Read the model definition and answer for the solid it produces. Units are mm, in the model's axes. Face numbers are marked on the shaded views. A direction names the side the tool comes from. Give positions to 0.01 mm unless a question says otherwise; leave off trailing zeros. Order: outer loops, then holes, each group sorted by start corner. A loop starts at its lowest first (then second) coordinate and runs counter-clockwise, first axis right, second up. Notation, with made-up numbers: (-9.75, -40) - (42.25, -40) arc R16 ccw to (42.25, -29) - close; hole circle Ø3 at (82.25, -33). An arc over 180 degrees is marked (long way). Use a Markdown table: item, result. Add a question column.
1. A cutting plane is placed at B-B on x = -22.5. Determine the outline of the cut face in (y, z), and give its area (3 significant figures).
2. A cutting plane is placed at A-A on y = -28. Determine the outline of the cut face in (x, z), and give its area (3 significant figures).
3. For a pull along X with two mould halves and no side action, classify the marked faces 3, 4, 5 and 6 as released by +X, released by -X, zero draft, split by the parting line, or undercut.
4. Which of the six approach directions +Z, -Z, +X, -X, +Y, -Y give full straight-line access (tool end or side, diameter ignored) to the marked faces 1 and 2?
5. Consider L1, parallel to Z at x = -32, y = -68; L2, parallel to X at y = -28, z = 5. Determine where each line is inside the solid, lowest interval first.
6. A cutting plane is placed at C-C on z = -3.5. Determine the outline of the cut face in (x, y), and give its area (3 significant figures).
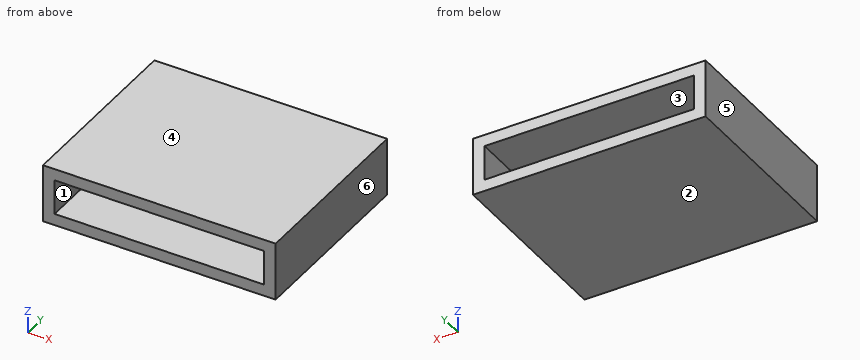
```python
from build123d import *

# Parameters (mm, degrees)
F2_DEPTH = 80


with BuildPart() as f2:
    # F1 (on Front) → F2 (new body)
    with BuildSketch(Plane.XZ):
        Polygon((50, 12.5), (0, 12.5), (0, 7.5), (45, 7.5), (45, -7.5), (0, -7.5), (0, -12.5), (50, -12.5), align=None)
    extrude(amount=F2_DEPTH)

    # F3: F2 across plane


with BuildPart() as f2_1:
    add(f2.part)
    add(f2.part.mirror(Plane.YZ))


solid = f2_1.part
```
Output values:
| question | item | result |
|---|---|---|
| 1 | outline | (-80, -12.5) - (0, -12.5) - (0, -7.5) - (-80, -7.5) - close; (-80, 7.5) - (0, 7.5) - (0, 12.5) - (-80, 12.5) - close |
| 1 | area | 800 mm² |
| 2 | outline | (-50, -12.5) - (50, -12.5) - (50, 12.5) - (-50, 12.5) - close; hole (-45, -7.5) - (45, -7.5) - (45, 7.5) - (-45, 7.5) - close |
| 2 | area | 1,150 mm² |
| 3 | face 3 | undercut |
| 3 | face 4 | zero draft |
| 3 | face 5 | released by -X |
| 3 | face 6 | released by +X |
| 4 | face 1 | +Y, -Y |
| 4 | face 2 | -Z, +X, -X, +Y, -Y |
| 5 | L1 | -12.5 to -7.5, 7.5 to 12.5 |
| 5 | L2 | -50 to -45, 45 to 50 |
| 6 | outline | (-50, -80) - (-45, -80) - (-45, 0) - (-50, 0) - close; (45, -80) - (50, -80) - (50, 0) - (45, 0) - close |
| 6 | area | 800 mm² |
